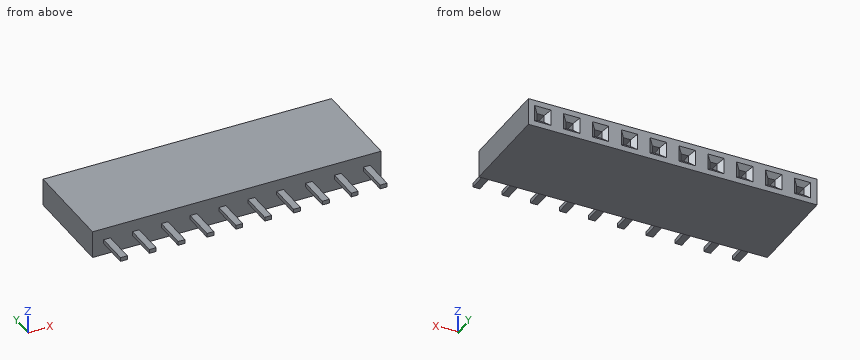
```python
from build123d import *

# Parameters (mm, degrees)
SKETCH1_W           = 38.1
SKETCH1_H           = 2.4
BOSS_EXTRUDE1_DEPTH = 8.5
SKETCH2_W           = 0.63
SKETCH2_H           = 0.63
CUT_EXTRUDE1_DEPTH  = 6.5
SKETCH3_W           = 0.6
SKETCH3_H           = 0.35
BOSS_EXTRUDE2_DEPTH = 2.9
CHAMFER1_SIZE       = 0.4
SKETCH4_W           = 19.378829163
SKETCH4_H           = 4.471478983
CUT_EXTRUDE2_DEPTH  = 23.232914789


with BuildPart() as part:
    # Sketch1 → Boss-Extrude1 (new body)
    with BuildSketch(Plane(origin=(0, 0, 0), x_dir=(1, 0, 0), z_dir=(0, 1, 0))):
        Rectangle(SKETCH1_W, SKETCH1_H)
    extrude(amount=BOSS_EXTRUDE1_DEPTH)

    # Sketch2 → Cut-Extrude1 (cut)
    with BuildSketch(Plane(origin=(0, 8.5, 0), x_dir=(1, 0, 0), z_dir=(0, 1, 0))):
        with Locations((-15.24, 0)):
            Rectangle(SKETCH2_W, SKETCH2_H)
        with Locations((-17.78, 0)):
            Rectangle(SKETCH2_W, SKETCH2_H)
        with Locations((-12.7, 0)):
            Rectangle(SKETCH2_W, SKETCH2_H)
        with Locations((-10.16, 0)):
            Rectangle(SKETCH2_W, SKETCH2_H)
        with Locations((-7.62, 0)):
            Rectangle(SKETCH2_W, SKETCH2_H)
        with Locations((-5.08, 0)):
            Rectangle(SKETCH2_W, SKETCH2_H)
        with Locations((-2.54, 0)):
            Rectangle(SKETCH2_W, SKETCH2_H)
        Rectangle(SKETCH2_W, SKETCH2_H)
        with Locations((2.54, 0)):
            Rectangle(SKETCH2_W, SKETCH2_H)
        with Locations((5.08, 0)):
            Rectangle(SKETCH2_W, SKETCH2_H)
        with Locations((7.62, 0)):
            Rectangle(SKETCH2_W, SKETCH2_H)
        with Locations((10.16, 0)):
            Rectangle(SKETCH2_W, SKETCH2_H)
        with Locations((12.7, 0)):
            Rectangle(SKETCH2_W, SKETCH2_H)
        with Locations((15.24, 0)):
            Rectangle(SKETCH2_W, SKETCH2_H)
        with Locations((17.78, 0)):
            Rectangle(SKETCH2_W, SKETCH2_H)
    extrude(amount=-CUT_EXTRUDE1_DEPTH, mode=Mode.SUBTRACT)

    # Sketch3 → Boss-Extrude2 (add)
    with BuildSketch(Plane.XZ):
        with Locations((-15.24, 0)):
            Rectangle(SKETCH3_W, SKETCH3_H)
        with Locations((-17.78, 0)):
            Rectangle(SKETCH3_W, SKETCH3_H)
        with Locations((-12.7, 0)):
            Rectangle(SKETCH3_W, SKETCH3_H)
        with Locations((-10.16, 0)):
            Rectangle(SKETCH3_W, SKETCH3_H)
        with Locations((-7.62, 0)):
            Rectangle(SKETCH3_W, SKETCH3_H)
        with Locations((-5.08, 0)):
            Rectangle(SKETCH3_W, SKETCH3_H)
        with Locations((-2.54, 0)):
            Rectangle(SKETCH3_W, SKETCH3_H)
        Rectangle(SKETCH3_W, SKETCH3_H)
        with Locations((2.54, 0)):
            Rectangle(SKETCH3_W, SKETCH3_H)
        with Locations((5.08, 0)):
            Rectangle(SKETCH3_W, SKETCH3_H)
        with Locations((7.62, 0)):
            Rectangle(SKETCH3_W, SKETCH3_H)
        with Locations((10.16, 0)):
            Rectangle(SKETCH3_W, SKETCH3_H)
        with Locations((12.7, 0)):
            Rectangle(SKETCH3_W, SKETCH3_H)
        with Locations((15.24, 0)):
            Rectangle(SKETCH3_W, SKETCH3_H)
        with Locations((17.78, 0)):
            Rectangle(SKETCH3_W, SKETCH3_H)
    extrude(amount=BOSS_EXTRUDE2_DEPTH)

    # Chamfer1
    chamfer1_edges = [part.edges().sort_by_distance(p)[0] for p in [
        (2.855, 8.5, 0),
        (2.54, 8.5, -0.315),
        (2.225, 8.5, 0),
        (2.54, 8.5, 0.315),
        (5.395, 8.5, 0),
        (5.08, 8.5, -0.315),
        (4.765, 8.5, 0),
        (5.08, 8.5, 0.315),
        (7.935, 8.5, 0),
        (7.62, 8.5, -0.315),
        (7.305, 8.5, 0),
        (7.62, 8.5, 0.315),
        (10.475, 8.5, 0),
        (10.16, 8.5, -0.315),
        (9.845, 8.5, 0),
        (10.16, 8.5, 0.315),
        (13.015, 8.5, 0),
        (12.7, 8.5, -0.315),
        (12.385, 8.5, 0),
        (12.7, 8.5, 0.315),
        (15.555, 8.5, 0),
        (15.24, 8.5, -0.315),
        (14.925, 8.5, 0),
        (15.24, 8.5, 0.315),
        (18.095, 8.5, 0),
        (17.78, 8.5, -0.315),
        (17.465, 8.5, 0),
        (17.78, 8.5, 0.315),
        (-17.465, 8.5, 0),
        (-17.78, 8.5, -0.315),
        (-18.095, 8.5, 0),
        (-17.78, 8.5, 0.315),
        (-14.925, 8.5, 0),
        (-15.24, 8.5, -0.315),
        (-15.555, 8.5, 0),
        (-15.24, 8.5, 0.315),
        (-12.385, 8.5, 0),
        (-12.7, 8.5, -0.315),
        (-13.015, 8.5, 0),
        (-12.7, 8.5, 0.315),
        (-9.845, 8.5, 0),
        (-10.16, 8.5, -0.315),
        (-10.475, 8.5, 0),
        (-10.16, 8.5, 0.315),
        (-7.305, 8.5, 0),
        (-7.62, 8.5, -0.315),
        (-7.935, 8.5, 0),
        (-7.62, 8.5, 0.315),
        (-4.765, 8.5, 0),
        (-5.08, 8.5, -0.315),
        (-5.395, 8.5, 0),
        (-5.08, 8.5, 0.315),
        (-2.225, 8.5, 0),
        (-2.54, 8.5, -0.315),
        (-2.855, 8.5, 0),
        (-2.54, 8.5, 0.315),
        (0.315, 8.5, 0),
        (0, 8.5, -0.315),
        (-0.315, 8.5, 0),
        (0, 8.5, 0.315),
    ]]
    chamfer(chamfer1_edges, length=CHAMFER1_SIZE)

    # Sketch4 → Cut-Extrude2 (cut, through all)
    with BuildSketch(Plane(origin=(0, 8.5, 0), x_dir=(1, 0, 0), z_dir=(0, 1, 0))):
        with Locations((16.039414582, -0.096925096)):
            Rectangle(SKETCH4_W, SKETCH4_H)
    extrude(amount=-CUT_EXTRUDE2_DEPTH, mode=Mode.SUBTRACT)


solid = part.part
```
CAD build for the part. Positions are in the model's coordinates, mm. Round coordinates to 2 decimals unless told otherwise and drop trailing zeros. Order: outer loops, then holes, each group sorted by start corner. A loop starts at its lowest first (then second) coordinate and runs counter-clockwise, first axis right, second up. Notation, with made-up numbers: (73.5, -25) - (89.5, -25) arc R28 ccw to (89.5, 12) - close; hole circle Ø10 at (-14, 85.5). An arc over 180 degrees is marked (long way). Answer as CSV lines item,"result". Start each with the question number.
1. Saw through at A-A, the plane x = 2.5. Write the cut outline in (y, z) (3 decimals).
2. Pin check, flat tip, straight feed: pin 1 (0.7 mm diameter, centred on x = -7.5, y = -1, fed in from +Z) (3 decimals). Stop position of the tip, or through.
3. Drill centre lines: L1, parallel to Z at x = -15, y = 5 (3 decimals); L2, parallel to Y at x = -0.25, z = -0.95; L3, parallel to Y at x = -8.25, z = -0.55 (3 decimals). Where is each one in solid material? Low to high. Write a range as [from, to].
4. Saw through at B-B, the plane y = -2. Count the separate pieces of the cut face and the enclosed holes in it, and give its area (3 significant figures).
Model answer:
1,outline,"(-2.9, -0.175) - (0, -0.175) - (0, -1.2) - (8.5, -1.2) - (8.5, -0.715) - (8.1, -0.315) - (2, -0.315) - (2, 0.315) - (8.1, 0.315) - (8.5, 0.715) - (8.5, 1.2) - (0, 1.2) - (0, 0.175) - (-2.9, 0.175) - close"
2,pin 1,"stops at z = 0.175"
3,L1,"z = [-1.2, -0.315], [0.315, 1.2]"
3,L2,"y = [0, 8.5]"
3,L3,"y = [0, 8.415]"
4,separate pieces,"10"
4,enclosed holes,"0"
4,area,"2.10 mm²"
